```python
from build123d import *

# Parameters (mm, degrees)
F1_DEPTH = 15.875


# Not quite as in the source:
# - ends of sketch curves that miss each other by under 0.0002 mm in the source are joined
# - the program builds the solid bodies; features that only make, move or delete a surface that nothing else refers to are left out


with BuildPart() as f1:
    # F0 (on Top) → F1 (new body)
    with BuildSketch(Plane.XY):
        with BuildLine():
            Line((-11.1125005688, -19.05), (11.1124994312, -19.05))
            ThreePointArc((11.1124994312, -19.05), (14.4800954095, -17.6550961124), (15.8749994312, -14.2875001896))
            Line((15.8749994312, -14.2875001896), (15.874999684, -7.9375001896))
            ThreePointArc((15.874999684, -7.9375001896), (14.4800957964, -4.5699040216), (11.112499684, -3.175))
            ThreePointArc((11.112499684, -3.175), (14.4800960416, -1.7800961124), (15.8750000632, 1.5874998104))
            Line((15.8750000632, 1.5874998104), (15.8750007584, 19.05))
            Line((15.8750007584, 19.05), (15.8750007584, 23.8125))
            ThreePointArc((15.8750007584, 23.8125), (14.4800968038, 27.1800960454), (11.1125007584, 28.575))
            Line((11.1125007584, 28.575), (-11.1124992416, 28.575))
            ThreePointArc((-11.1124992416, 28.575), (-14.480095287, 27.1800960454), (-15.8749992416, 23.8125))
            Line((-15.8749992416, 23.8125), (-15.8749992416, 19.05))
            Line((-15.8749992416, 19.05), (-15.8750005688, -14.2874998104))
            ThreePointArc((-15.8750005688, -14.2874998104), (-14.4800966813, -17.6550959784), (-11.1125005688, -19.05))
        make_face()
        with BuildLine():
            Line((-12.7, -6.35), (-12.7, -4.7625))
            ThreePointArc((-12.7, -4.7625), (-12.2350320151, -5.8850320151), (-11.1125, -6.35))
            Line((-11.1125, -6.35), (11.1125, -6.35))
            ThreePointArc((11.1125, -6.35), (12.2350320151, -6.8149679849), (12.7, -7.9375))
            Line((12.7, -7.9375), (12.7, -14.2875))
            ThreePointArc((12.7, -14.2875), (12.2350320151, -15.4100320151), (11.1125, -15.875))
            Line((11.1125, -15.875), (-11.1125, -15.875))
            ThreePointArc((-11.1125, -15.875), (-12.2350320151, -15.4100320151), (-12.7, -14.2875))
            Line((-12.7, -14.2875), (-12.7, -6.35))
        make_face(mode=Mode.SUBTRACT)
        with BuildLine():
            ThreePointArc((-12.7, -1.5875), (-12.2350320151, -2.7100320151), (-11.1125, -3.175))
            ThreePointArc((-11.1125, -3.175), (-12.2350320151, -3.6399679849), (-12.7, -4.7625))
            Line((-12.7, -4.7625), (-12.7, -3.175))
            Line((-12.7, -3.175), (-12.7, -1.5875))
        make_face(mode=Mode.SUBTRACT)
        with BuildLine():
            ThreePointArc((-11.1125, 0), (-12.2350320151, -0.4649679849), (-12.7, -1.5875))
            Line((-12.7, -1.5875), (-12.7, 0))
            Line((-12.7, 0), (-12.7, 23.8125))
            ThreePointArc((-12.7, 23.8125), (-12.2350320151, 24.9350320151), (-11.1125, 25.4))
            Line((-11.1125, 25.4), (11.1125, 25.4))
            ThreePointArc((11.1125, 25.4), (12.2350320151, 24.9350320151), (12.7, 23.8125))
            Line((12.7, 23.8125), (12.7, 1.5875))
            ThreePointArc((12.7, 1.5875), (12.2350320151, 0.4649679849), (11.1125, 0))
            Line((11.1125, 0), (-11.1125, 0))
        make_face(mode=Mode.SUBTRACT)
        with BuildLine():
            Line((-12.7, -3.175), (-11.1125, -3.175))
            ThreePointArc((-11.1125, -3.175), (-12.2350320151, -2.7100320151), (-12.7, -1.5875))
            Line((-12.7, -1.5875), (-12.7, -3.175))
        make_face()
        with BuildLine():
            ThreePointArc((-12.7, -4.7625), (-12.2350320151, -3.6399679849), (-11.1125, -3.175))
            Line((-11.1125, -3.175), (-12.7, -3.175))
            Line((-12.7, -3.175), (-12.7, -4.7625))
        make_face()
    extrude(amount=F1_DEPTH)


solid = f1.part
```
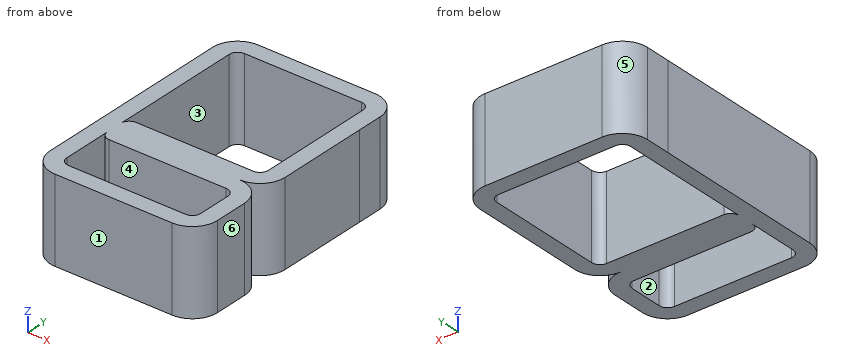
For this review, take the finished solid that the model builds, in its own axes (mm). Face numbers are marked on the shaded views. A direction names the side the tool comes from. Give positions to 0.01 mm unless a question says otherwise; leave off trailing zeros. Loops run counter-clockwise (first coordinate to the right, second up) from the corner with the lowest first, then second, coordinate; pieces in that order, holes last. Notation, with made-up numbers: M -0.75,40.5 L 12.25,40.5 A22 cw 12.25,47.5 Z; hole C 59,50 d5. An arc over 180 degrees is marked long. One line per item, written item: value. Start each with the question number.
Q1. Add section A-A (x = 7). Give the boundary of the cut face in (y, z) (3 decimals).
Q2. For L1, parallel to Y at x = 4, z = 4 (3 decimals); L2, parallel to X at y = 16.5, z = 3.5 (3 decimals); L3, parallel to Y at x = -11.5, z = 6, list the stretches that pass through material, from the lowest coordinate up.
Q3. Clearance check with a flat-ended pin moving along its axis: pin 1 Ø8 at (x, y) = (-5, -3) entering from -Z. State where the tip first meets the part, or that it passes through.
Q4. Machinability: for the marked faces 1 and 2, which of the approach directions +Z, -Z, +X, -X, +Y, -Y give a long, thin tool a straight path to every point of the face, cutting with its end or side? Answer none if there is none.
Q5. Draft analysis for pull direction Y (two halves, no side actions). For the marked faces 3, 4, 5 and 6, state which applies: released by +Y, released by -Y, zero draft, split by the parting line, or undercut.
Q6. Add section C-C (z = 10.5). Count the separate pieces of the cut face and the enclosed holes in it, and give its area (3 significant figures).
Q7. Add section B-B (y = 15). Give the boundary of the cut face in (x, z) (3 decimals).
Reply:
1. outline: M -19.05,0 L -15.875,0 L -15.875,15.875 L -19.05,15.875 Z; M -6.35,0 L 0,0 L 0,15.875 L -6.35,15.875 Z; M 25.4,0 L 28.575,0 L 28.575,15.875 L 25.4,15.875 Z
2. L1: -19.05 to -15.875, -6.35 to 0, 25.4 to 28.575
2. L2: -15.875 to -12.7, 12.7 to 15.875
2. L3: -19.03 to -15.83, -6.3 to -0.05, 25.35 to 28.56
3. pin 1: z = 0
4. face 1: +Z, -Z, +X, -X, -Y
4. face 2: +Z, -Z
5. face 3: undercut
5. face 4: undercut
5. face 5: released by +Y
5. face 6: zero draft
6. separate pieces: 1
6. enclosed holes: 2
6. area: 598 mm²
7. outline: M -15.875,0 L -12.7,0 L -12.7,15.875 L -15.875,15.875 Z; M 12.7,0 L 15.875,0 L 15.875,15.875 L 12.7,15.875 Z
